Design review of the part built by this model. Coordinates are the model's own, in mm. A direction names the side the tool comes from. Round coordinates to 2 decimals unless told otherwise and drop trailing zeros. Write each loop counter-clockwise with the first axis right and the second up, starting at its lowest first coordinate (ties: lowest second). Pieces come first, ordered by that corner, then holes. Notation, with made-up numbers: (60.25, 60) -> (95.25, 60) arc R28 ccw to (95.25, 81) -> close; hole circle Ø8 at (-19, 38.5). An arc over 180 degrees is marked (long way). Write item = value, one per line. Start each with the question number.
Item 1: Add section A-A, the plane x = 0. State the section outline as (y, z) points (3 decimals).
Item 2: Mouldability with a two-part tool opening along Y and no side actions: class faces 1 (the flat face through (-5.35, 3.03, -32.54)), 2 (the flat face through (5, 0, 35.5)), 3 (the flat face through (0, -9.525, 0)) as released by +Y, released by -Y, zero draft, split by the parting line, or undercut.
Item 3: For pin 1 Ø3 at (x, z) = (8, -1) entering from +Y; pin 2 Ø3 at (x, y) = (-0.5, -8.5) entering from +Z; pin 3 Ø1.8 at (x, z) = (-1.5, -31.5) entering from -Y (3 decimals), all flat-tipped, find the tip position at first contact; note any pin that passes through.
Item 4: Machinability: for faces 4 (the flat face through (5.3, 3.12, -32.54)), 5 (the flat face through (-8.287, -4.696, -0.497)), 6 (the flat face through (8.287, 4.696, -0.497)), which of the approach directions +Z, -Z, +X, -X, +Y, -Y give a long, thin tool a straight path to every point of the face, cutting with its end or side? Answer none if there is none.
Item 5: Add section B-B, the plane z = -11. State the section outline as (x, y) points (3 decimals).
Item 6: To check wall thickness, follow L1, parallel to Y at x = 0, z = -36; L2, parallel to Z at x = 6.75, y = 0; L3, parallel to Y at x = 0.75, z = -17.5 (3 decimals). State the ranges of each line that lie inside material, in increasing order.
from build123d import *

# Parameters (mm, degrees)
BOSS_EXTRUDE1_DEPTH      = 35.5
BOSS_EXTRUDE1_DEPTH_BACK = 35.5
CUT_EXTRUDE1_DEPTH       = 6
SKETCH4_R                = 11.5
SKETCH4_R_2              = 8.5
BOSS_EXTRUDE3_DEPTH      = 2
SKETCH5_R                = 4
BOSS_EXTRUDE4_DEPTH      = 8


with BuildPart() as part:
    # Sketch1 → Boss-Extrude1 (new, two sides: drawn at the far end of the back side and taken through both)
    with BuildSketch(Plane.XY.offset(-BOSS_EXTRUDE1_DEPTH_BACK)):
        Polygon((10.998522628, 0), (5.499261314, 9.525), (-5.499261314, 9.525), (-10.998522628, 0), (-5.499261314, -9.525), (5.499261314, -9.525), align=None)
    extrude(amount=BOSS_EXTRUDE1_DEPTH + BOSS_EXTRUDE1_DEPTH_BACK)

    # Sketch2 → Cut-Extrude1 (cut)
    with BuildSketch(Plane(origin=(0, 0, -35.5), x_dir=(-1, 0, 0), z_dir=(0, 0, -1))):
        Polygon((7.101408311, 0), (3.550704156, 6.15), (-3.550704156, 6.15), (-7.101408311, 0), (-3.550704156, -6.15), (3.550704156, -6.15), align=None)
    extrude(amount=-CUT_EXTRUDE1_DEPTH, mode=Mode.SUBTRACT)

    # Sketch4 → Boss-Extrude3 (add)
    with BuildSketch(Plane(origin=(0, 0, -35.5), x_dir=(-1, 0, 0), z_dir=(0, 0, -1))):
        Circle(SKETCH4_R)
        Circle(SKETCH4_R_2, mode=Mode.SUBTRACT)
    extrude(amount=BOSS_EXTRUDE3_DEPTH)

    # Sketch5 → Boss-Extrude4 (add)
    with BuildSketch(Plane.XY.offset(35.5)):
        Circle(SKETCH5_R)
    extrude(amount=BOSS_EXTRUDE4_DEPTH)


solid = part.part
Result set:
q1.outline = (-11.5, -37.5) -> (-8.5, -37.5) -> (-8.5, -35.5) -> (-6.15, -35.5) -> (-6.15, -29.5) -> (6.15, -29.5) -> (6.15, -35.5) -> (8.5, -35.5) -> (8.5, -37.5) -> (11.5, -37.5) -> (11.5, -35.5) -> (9.525, -35.5) -> (9.525, 35.5) -> (4, 35.5) -> (4, 43.5) -> (-4, 43.5) -> (-4, 35.5) -> (-9.525, 35.5) -> (-9.525, -35.5) -> (-11.5, -35.5) -> close
q2.face_1 = undercut
q2.face_2 = zero draft
q2.face_3 = released by -Y
q3.pin_1 = 7.79
q3.pin_2 = 35.5
q3.pin_3 = -9.525
q4.face_4 = -Z
q4.face_5 = +Z, -X, -Y
q4.face_6 = +Z, +X, +Y
q5.outline = (-10.999, 0) -> (-5.499, -9.525) -> (5.499, -9.525) -> (10.999, 0) -> (5.499, 9.525) -> (-5.499, 9.525) -> close
q6.L1 = -11.5 to -8.5, 8.5 to 11.5
q6.L2 = -29.5 to 35.5
q6.L3 = -9.525 to 9.525
